Source: CAD feature listing. Evaluate the final solid. Frame: model axes, mm. A direction names the side the tool comes from. Give positions to 0.01 mm unless a question says otherwise; leave off trailing zeros. Order: outer loops, then holes, each group sorted by start corner. A loop starts at its lowest first (then second) coordinate and runs counter-clockwise, first axis right, second up. Notation, with made-up numbers: (-40, 41.25) - (5, 41.25) arc R24 ccw to (5, 76.25) - close; hole circle Ø8 at (-24, 42.25). An arc over 180 degrees is marked (long way). Write each question's results on one line, items separated by ' | '. Start each with the question number.
Item 1: Section B-B on z = 264. Output: boundary loops of the cut face in (x, y).
Item 2: Line query: line 1 along Z through (x, y) = (479.5, -10); line 2 along X through (y, z) = (-2, 1226); line 3 along Y through (x, z) = (528.5, 94). Output: solid intervals per line, ascending.
Item 3: Section D-D on x = 237.5. Output: boundary loops of the cut face in (y, z).
Item 4: Contact query for flat-ended pins moving along their axis: pin 1 Ø10 at (y, z) = (16.5, 339) entering from -X; pin 2 Ø10 at (x, y) = (33.5, 10.5) entering from +Z; pin 3 Ø12 at (x, z) = (575.5, 547.5) entering from -Y. Output: stop coordinate, or through.
Item 5: Section A-A on x = 722. Output: boundary loops of the cut face in (y, z), and give its area (3 significant figures).
Item 6: Mould query, pull axis X, two halves, no side actions, for faces 3 (the flat face through (776, 0, 1157)), 4 (the flat face through (385, 0, 1434)). Classes: released by +X, released by -X, zero draft, split by the parting line, or undercut.
Item 7: Section C-C on y = 19. Output: boundary loops of the cut face in (x, z).
Item 8: Set-up query: faces 1 (the flat face through (776, -13.97, 1157)), 2 (the flat face through (385, 0, 533)). Return all of +Z, -Z, +X, -X, +Y, -Y with unobstructed straight access to the full face (end or side cutting, diameter ignored); none if empty.
```python
from build123d import *

# Parameters (mm, degrees)
F0_W     = 762
F0_H     = 1905
F0_W_2   = 558.8
F0_H_2   = 850.9
F0_H_3   = 749.3
F1_DEPTH = 12.7
F3_DEPTH = 13.97
F4_W     = 762
F4_H     = 1905
F5_DEPTH = 25.4


with BuildPart() as f1:
    # F0 (on Front) → F1 (new body)
    with BuildSketch(Plane.XZ):
        with Locations((381, 952.5)):
            Rectangle(F0_W, F0_H)
        with Locations((381, 527.05)):
            Rectangle(F0_W_2, F0_H_2, mode=Mode.SUBTRACT)
        with Locations((381, 1428.75)):
            Rectangle(F0_W_2, F0_H_3, mode=Mode.SUBTRACT)
    extrude(amount=F1_DEPTH)

    # F2 (on face) → F3 (join)
    with BuildSketch(Plane(origin=(0, 0, 0), x_dir=(-1, 0, 0), z_dir=(0, 1, 0))):
        Polygon((0, 1905), (0, 0), (101.6, 0), (101.6, 2006.6), (-863.6, 2006.6), (-863.6, 0), (-762, 0), (-762, 1905), align=None)
    extrude(amount=-F3_DEPTH)

    # F4 (on face) → F5 (join)
    with BuildSketch(Plane(origin=(0, 0, 0), x_dir=(-1, 0, 0), z_dir=(0, 1, 0))):
        with Locations((-381, 952.5)):
            Rectangle(F4_W, F4_H)
    extrude(amount=F5_DEPTH)


solid = f1.part
```
Evaluation:
1) outline: (-101.6, -13.97) - (0, -13.97) - (0, -12.7) - (101.6, -12.7) - (101.6, 0) - (660.4, 0) - (660.4, -12.7) - (762, -12.7) - (762, -13.97) - (863.6, -13.97) - (863.6, 0) - (762, 0) - (762, 25.4) - (0, 25.4) - (0, 0) - (-101.6, 0) - close
2) line 1: z = 0 to 101.6, 952.5 to 1054.1, 1803.4 to 2006.6 | line 2: x = -101.6 to 101.6, 660.4 to 863.6 | line 3: y = -12.7 to 25.4
3) outline: (-13.97, 1905) - (-12.7, 1905) - (-12.7, 1803.4) - (0, 1803.4) - (0, 1054.1) - (-12.7, 1054.1) - (-12.7, 952.5) - (0, 952.5) - (0, 101.6) - (-12.7, 101.6) - (-12.7, 0) - (25.4, 0) - (25.4, 1905) - (0, 1905) - (0, 2006.6) - (-13.97, 2006.6) - close
4) pin 1: stops at x = 0 | pin 2: stops at z = 1905 | pin 3: stops at y = 0
5) outline: (-13.97, 1905) - (-12.7, 1905) - (-12.7, 0) - (25.4, 0) - (25.4, 1905) - (0, 1905) - (0, 2006.6) - (-13.97, 2006.6) - close | area: 74,000 mm^2
6) face 3: zero draft | face 4: undercut
7) outline: (0, 0) - (762, 0) - (762, 1905) - (0, 1905) - close
8) face 1: +Z, -Z, +X, -X, -Y | face 2: -Y
